from build123d import *

# Parameters (mm, degrees)
F0_R     = 44.45
F1_DEPTH = 3.81
F2_R     = 38.1
F3_DEPTH = 9.525
F5_D     = 6.985


with BuildPart() as f1:
    # F0 (on Top) → F1 (new body)
    with BuildSketch(Plane.XY):
        Circle(F0_R)
    extrude(amount=F1_DEPTH)

    # F2 (on face) → F3 (join)
    with BuildSketch(Plane.XY.offset(3.81)):
        Circle(F2_R)
    extrude(amount=F3_DEPTH)

    # F5 (through all)
    with Locations(Plane.XY.offset(13.335)):
        with Locations((0, 0)):
            Hole(F5_D / 2)


solid = f1.part
Geometry: final body of the model. Coordinates: model frame, mm. A direction names the side the tool comes from. Give positions to 0.01 mm unless a question says otherwise; leave off trailing zeros. Order: outer loops, then holes, each group sorted by start corner. A loop starts at its lowest first (then second) coordinate and runs counter-clockwise, first axis right, second up. Notation, with made-up numbers: (-39, 8.5) - (-24, 8.5) arc R18 ccw to (-24, 32.5) - close; hole circle Ø10 at (-9.5, -10.5). An arc over 180 degrees is marked (long way). Use CSV: the item, a comma, the result in double quotes.
1. Mould query, pull axis X, two halves, no side actions, for faces 3 (the face through (-1, -9, 0)), 4 (the face through (-30.235, -23.183, 8.506)), 5 (the face through (0.455, 3.463, 6.574)). Classes: +X half, -X half, draft (parallel to the pull), parting line (faces both ways), or undercut.
Answers below:
face 3,"draft"
face 4,"parting line"
face 5,"undercut"
2. Section query D-D (y = -31.5). Output: boundary loops of the cut face in (x, z) (3 decimals).
Answers below:
outline,"(-31.362, 0) - (31.362, 0) - (31.362, 3.81) - (21.433, 3.81) - (21.433, 13.335) - (-21.433, 13.335) - (-21.433, 3.81) - (-31.362, 3.81) - close"
3. Contact query for flat-ended pins moving along their axis: pin 1 (1.5 mm diameter, centred on y = -25, z = 9.5, fed in from -X); pin 2 (3 mm diameter, centred on x = -7.5, z = 9, fed in from +Y); pin 3 (2 mm diameter, centred on y = 24.5, z = 2, fed in from +X). Output: stop coordinate, or through.
Answers below:
pin 1,"x = -29.39"
pin 2,"y = 37.62"
pin 3,"x = 37.73"
4. Material intervals for line 1 along Y through (x, z) = (0, 8.5); line 2 along Y through (x, z) = (0, 3.5); line 3 along Z through (x, y) = (37.5, 19), sorted ascending. Write a range as from..to.
Answers below:
line 1,"-38.1..-3.49, 3.49..38.1"
line 2,"-44.45..-3.49, 3.49..44.45"
line 3,"0..3.81"
5. Section query C-C (z = 8.5). Output: boundary loops of the cut face in (x, y) (1 decimal), plus the area to 3 significant figures.
Answers below:
outline,"circle Ø76.2 at (0, 0); hole circle Ø7 at (0, 0)"
area,"4,520 mm2"
6. Access query for faces 1 (the face through (8, 1, 13.335)), 2 (the face through (33, 20, 3.81)). Directions: +Z, -Z, +X, -X, +Y, -Y. A direction counts if a zero-diameter tool reaches every point of the face in a straight line with its end or side. Return the directions, or none.
Answers below:
face 1,"+Z, +X, -X, +Y, -Y"
face 2,"+Z"
